Could you check a few things on this model? Use its own coordinates, in mm. Give positions to 0.01 mm unless a question says otherwise; leave off trailing zeros. Loops run counter-clockwise (first coordinate to the right, second up) from the corner with the lowest first, then second, coordinate; pieces in that order, holes last. Notation, with made-up numbers: (52, -0.5) - (101, -0.5) arc R14 ccw to (101, 17.5) - close; hole circle Ø3 at (-17.5, 88). An arc over 180 degrees is marked (long way). One line per item, written item: value. Start each with the question number.
Q1. I want a section at C-C (x = -40). Please give me the cut outline in (y, z).
Q2. I'm going to push flat-ended pins straight in: P1, Ø1.5, axis at x = -48, y = -1, coming from the +Z side; P2, Ø8, axis at x = 21.5, z = 37, coming from the +Y side. Where does each tip first touch, or does it pass through?
Q3. I want a section at D-D (x = 50.5). Please give me the cut outline in (y, z), then the cut area to 3 significant figures.
Q4. I want a section at B-B (z = 30.5). Please give me the cut outline in (x, y).
Q5. I want a section at A-A (y = 0.9). Please give me the cut outline in (x, z), then the cut area to 3 significant figures.
Q6. If I drill on line 1 (X direction, y = -1.1, z = -13); line 2 (Z direction, x = 12, y = 0.9); line 3 (Z direction, x = -43, y = -0.65), over which ranges is the centre line in solid material (lowest first)? Write a range as from..to.
```python
from build123d import *

# Parameters (mm, degrees)
SKETCH1_R           = 60
BOSS_EXTRUDE1_DEPTH = 1.5
CUT_EXTRUDE3_START  = -4
CUT_EXTRUDE3_DEPTH  = 5
CIRPATTERN1_COUNT   = 4


with BuildPart() as part:
    # Sketch1 → Boss-Extrude1 (new body, symmetric)
    with BuildSketch(Plane(origin=(0, 0, 0), x_dir=(1, 0, 0), z_dir=(0, 1, 0))):
        Circle(SKETCH1_R)
    extrude(amount=BOSS_EXTRUDE1_DEPTH, both=True)

    # Sketch4 → Cut-Extrude3 (cut)
    with BuildSketch(Plane(origin=(0, 1.5, 0), x_dir=(1, 0, 0), z_dir=(0, 1, 0)).offset(CUT_EXTRUDE3_START)):
        Polygon((9.545941546, 44.901280605), (44.901280605, 9.545941546), (47.022600949, 11.66726189), (11.66726189, 47.022600949), align=None)
    cut_extrude3 = extrude(amount=CUT_EXTRUDE3_DEPTH, mode=Mode.SUBTRACT)

    # CirPattern1: Cut-Extrude3 ×4 about axis
    cirpattern1_axis = Axis((0, 0, 0), (0, 1, 0))
    for i in range(1, CIRPATTERN1_COUNT):
        add(cut_extrude3.rotate(cirpattern1_axis, i * 360 / CIRPATTERN1_COUNT), mode=Mode.SUBTRACT)


solid = part.part
```
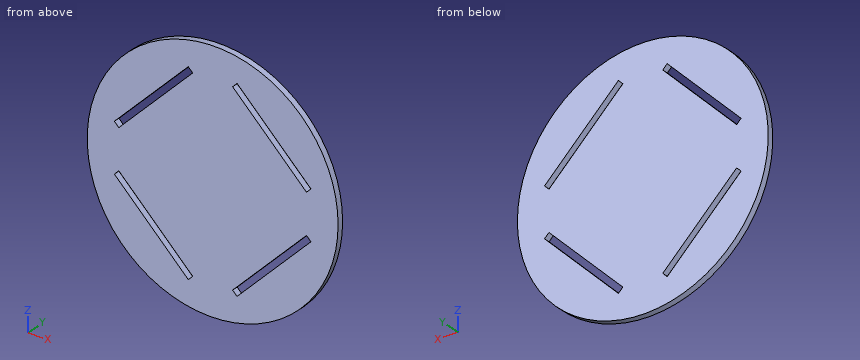
Worked answers:
1. outline: (-1.5, -44.72) - (1.5, -44.72) - (1.5, -18.69) - (-1.5, -18.69) - close; (-1.5, -14.45) - (1.5, -14.45) - (1.5, 14.45) - (-1.5, 14.45) - close; (-1.5, 18.69) - (1.5, 18.69) - (1.5, 44.72) - (-1.5, 44.72) - close
2. P1: stops at z = 36.98
2. P2: stops at y = 1.5
3. outline: (-1.5, -32.4) - (1.5, -32.4) - (1.5, 32.4) - (-1.5, 32.4) - close
3. area: 194 mm²
4. outline: (-51.67, -1.5) - (-28.19, -1.5) - (-28.19, 1.5) - (-51.67, 1.5) - close; (-23.95, -1.5) - (23.95, -1.5) - (23.95, 1.5) - (-23.95, 1.5) - close; (28.19, -1.5) - (51.67, -1.5) - (51.67, 1.5) - (28.19, 1.5) - close
5. outline: circle Ø120 at (0, 0); hole (-47.02, -11.67) - (-11.67, -47.02) - (-9.55, -44.9) - (-44.9, -9.55) - close; hole (-47.02, 11.67) - (-44.9, 9.55) - (-9.55, 44.9) - (-11.67, 47.02) - close; hole (9.55, -44.9) - (11.67, -47.02) - (47.02, -11.67) - (44.9, -9.55) - close; hole (9.55, 44.9) - (44.9, 9.55) - (47.02, 11.67) - (11.67, 47.02) - close
5. area: 10,700 mm²
6. line 1: x = -58.57..-45.69, -41.45..41.45, 45.69..58.57
6. line 2: z = -58.79..-46.69, -42.45..42.45, 46.69..58.79
6. line 3: z = -41.84..-15.69, -11.45..11.45, 15.69..41.84
